from build123d import *

# Parameters (mm, degrees)
SKETCH_R           = 17
PAD_DEPTH          = 10
POCKET_DEPTH       = 115.225233
POCKET_DEPTH_BACK  = 115.225233
POLARPATTERN_COUNT = 2
POLARPATTERN_ANGLE = 90


with BuildPart() as part:
    # Sketch → Pad (new body)
    with BuildSketch(Plane.XY):
        Circle(SKETCH_R)
    extrude(amount=PAD_DEPTH)

    # Sketch001 → Groove (revolve, cut)
    with BuildSketch(Plane.YZ):
        Polygon((0, 0), (0, 10), (16, 10), (15, 8.267949), (16, 1.5), (13.7, 1.5), (13.7, 2.7), (13.1, 2.7), (13.1, 1.5), (12.6, 1.5), (12.6, 0), align=None)
    revolve(axis=Axis((0, 0, 0), (0, 0, 1)), mode=Mode.SUBTRACT)

    # Sketch002 → Pocket (cut, two sides)
    with BuildSketch(Plane.XZ) as pocket_sk:
        with BuildLine():
            Line((-1.25, 10), (1.25, 10))
            Line((1.25, 10), (1.25, 5))
            ThreePointArc((-1.25, 5), (0, 3.75), (1.25, 5))
            Line((-1.25, 5), (-1.25, 10))
        make_face()
    pocket = extrude(amount=-POCKET_DEPTH, mode=Mode.SUBTRACT) + extrude(pocket_sk.sketch, amount=POCKET_DEPTH_BACK, mode=Mode.SUBTRACT)

    # PolarPattern: Pocket ×2 about axis
    polarpattern_axis = Axis((0, 0, 0), (0, 0, 1))
    for i in range(1, POLARPATTERN_COUNT):
        add(pocket.rotate(polarpattern_axis, i * POLARPATTERN_ANGLE / (POLARPATTERN_COUNT - 1)), mode=Mode.SUBTRACT)


solid = part.part
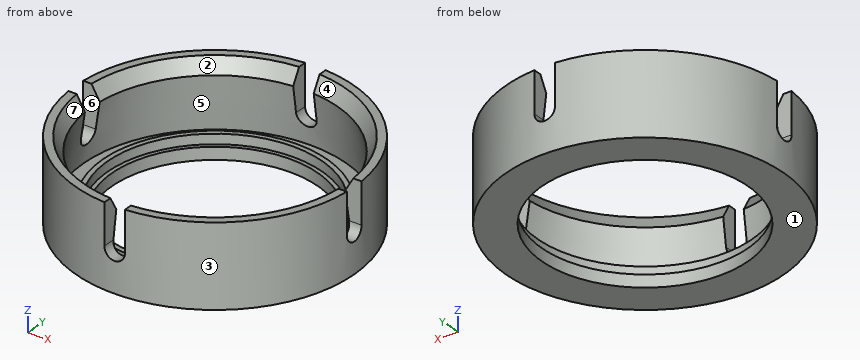
The listing builds one solid part. Answer for the finished solid, in the listing's coordinates (mm). Face numbers are marked on the shaded views. A direction names the side the tool comes from. Round coordinates to 2 decimals unless told otherwise and drop trailing zeros. Order: outer loops, then holes, each group sorted by start corner. A loop starts at its lowest first (then second) coordinate and runs counter-clockwise, first axis right, second up. Notation, with made-up numbers: (65, -9) -> (90, -9) arc R14 cw to (90, 8) -> close; hole circle Ø1 at (19.25, -16.75). An arc over 180 degrees is marked (long way). Put each result on its own line as item: value.
Q1. Section D-D, the plane z = 9.25 is taken. Write down the section's boundary in (x, y).
Results list:
outline: (-16.95, -1.25) arc R17 ccw to (-1.25, -16.95) -> (-1.25, -15.52) arc R15.57 cw to (-15.52, -1.25) -> close; (-16.95, 1.25) -> (-15.52, 1.25) arc R15.57 cw to (-1.25, 15.52) -> (-1.25, 16.95) arc R17 ccw to start; (1.25, -16.95) arc R17 ccw to (16.95, -1.25) -> (15.52, -1.25) arc R15.57 cw to (1.25, -15.52) -> close; (1.25, 15.52) arc R15.57 cw to (15.52, 1.25) -> (16.95, 1.25) arc R17 ccw to (1.25, 16.95) -> close
Q2. Which of the six approach directions +Z, -Z, +X, -X, +Y, -Y give full straight-line access (tool end or side, diameter ignored) to the marked faces 5, 6 and 7?
Results list:
face 5: none
face 6: +Z, +X, -X
face 7: +Z
Q3. Each of these flat-tipped pins is pushed along its axis until it touches: P1, Ø1, axis at x = 16, z = 8.5, coming from the -Y side; P2, Ø0.6, axis at y = 16, z = 8.5, coming from the +X side; P3, Ø1, axis at y = 15.5, z = 7, coming from the -X side. Where does it stop, or does it pass through?
Results list:
P1: y = -6.98
P2: x = 6.52
P3: x = -8
Q4. Determine the mould class of the marked faces 1, 2, 3 and 4 for opening direction X: pulls with the +X half, pulls with the -X half, needs draft (parallel to the pull), parting line crosses it, or undercut.
Results list:
face 1: needs draft
face 2: undercut
face 3: parting line crosses it
face 4: undercut
Q5. Section A-A, the plane z = 6.5 is taken. Write down the section's boundary in (x, y).
Results list:
outline: (-16.95, -1.25) arc R17 ccw to (-1.25, -16.95) -> (-1.25, -15.21) arc R15.26 cw to (-15.21, -1.25) -> close; (-16.95, 1.25) -> (-15.21, 1.25) arc R15.26 cw to (-1.25, 15.21) -> (-1.25, 16.95) arc R17 ccw to start; (1.25, -16.95) arc R17 ccw to (16.95, -1.25) -> (15.21, -1.25) arc R15.26 cw to (1.25, -15.21) -> close; (1.25, 15.21) arc R15.26 cw to (15.21, 1.25) -> (16.95, 1.25) arc R17 ccw to (1.25, 16.95) -> close
Q6. Consider line 1 along X through (y, z) = (0, 1.15); line 2 along X through (y, z) = (0, 1.8); line 3 along Y through (x, z) = (0, 2.35). Determine where each line is inside the solid, lowest interval first.
Results list:
line 1: -17 to -12.6, 12.6 to 17
line 2: -17 to -15.96, -13.7 to -13.1, 13.1 to 13.7, 15.96 to 17
line 3: -17 to -15.87, -13.7 to -13.1, 13.1 to 13.7, 15.87 to 17
Q7. Section B-B, the plane x = 0 is taken. Write down the section's boundary in (y, z), and give its area (3 significant figures).
Results list:
outline: (-17, 0) -> (-12.6, 0) -> (-12.6, 1.5) -> (-13.1, 1.5) -> (-13.1, 2.7) -> (-13.7, 2.7) -> (-13.7, 1.5) -> (-16, 1.5) -> (-15.67, 3.75) -> (-17, 3.75) -> close; (12.6, 0) -> (17, 0) -> (17, 3.75) -> (15.67, 3.75) -> (16, 1.5) -> (13.7, 1.5) -> (13.7, 2.7) -> (13.1, 2.7) -> (13.1, 1.5) -> (12.6, 1.5) -> close
area: 19.9 mm^2
